The model under review builds one solid part; all positions refer to its coordinate system, in mm. Coordinates: 2 decimals unless noted, no trailing zeros. Loops run counter-clockwise (first coordinate to the right, second up) from the corner with the lowest first, then second, coordinate; pieces in that order, holes last. Notation, with made-up numbers: (17, 89.25) -> (63, 89.25) arc R23 ccw to (63, 118.25) -> close; hole circle Ø11 at (19, -25.75). An arc over 180 degrees is marked (long way). One line per question, with ' | ' between items. Start each with the question number.
from build123d import *

# Parameters (mm, degrees)
F0_W     = 302
F0_H     = 600
F1_DEPTH = 21
F2_SIZE  = 20.99999
F3_W     = 21
F3_H     = 600
F4_DEPTH = 10
F5_W     = 302
F5_H     = 15
F6_DEPTH = 4
F7_W     = 281
F7_H     = 15
F8_DEPTH = 4


# Not quite as in the source:
# - a fillet or chamfer is up to 0.001 mm smaller than in the source, because OpenCascade refuses the exact size


with BuildPart() as f1:
    # F0 (on Front) → F1 (new body)
    with BuildSketch(Plane.XZ):
        with Locations((151, 300)):
            Rectangle(F0_W, F0_H)
    extrude(amount=-F1_DEPTH)

    # F2 (size 21 in the source; OpenCascade refuses exactly that, so slightly less here)
    f2_edges = [f1.edges().sort_by_distance(p)[0] for p in [
        (151, 0, 0),
        (151, 0, 600),
    ]]
    chamfer(f2_edges, length=F2_SIZE)

    # F3 (on face) → F4 (cut)
    with BuildSketch(Plane.XZ):
        with Locations((10.5, 300)):
            Rectangle(F3_W, F3_H)
    extrude(amount=-F4_DEPTH, mode=Mode.SUBTRACT)

    # F5 (on face) → F6 (cut)
    with BuildSketch(Plane.XZ):
        with Locations((151, 507.5)):
            Rectangle(F5_W, F5_H)
    extrude(amount=-F6_DEPTH, mode=Mode.SUBTRACT)

    # F7 (on face) → F8 (cut)
    with BuildSketch(Plane.XZ):
        with Locations((161.5, 335.5)):
            Rectangle(F7_W, F7_H)
        with Locations((161.5, 127.5)):
            Rectangle(F7_W, F7_H)
    extrude(amount=-F8_DEPTH, mode=Mode.SUBTRACT)


solid = f1.part
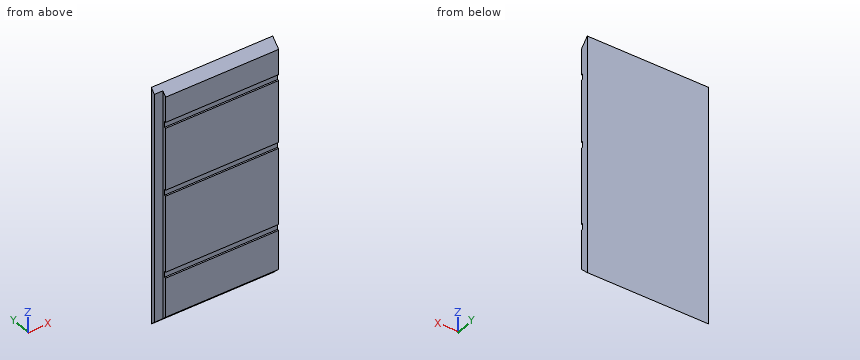
1) Insertion check: pin 1 Ø10 at (x, y) = (209, 10) entering from -Z; pin 2 Ø6 at (x, y) = (64, 17) entering from +Z; pin 3 Ø3 at (x, y) = (209.5, 3) entering from -Z. Each pin has a flat end and moves straight along its axis. Give the tip position at first contact, or say it passes through.
2) Consider section B-B, the plane z = 532. Write out the cut boundary in (x, y).
3) Wall thickness on L1, parallel to X at y = 3, z = 517; L2, parallel to Z at x = 220, y = 10; L3, parallel to Z at x = 272, y = 19.5: over which ranges is each line inside the solid? List them lowest first.
Filled sheet:
1) pin 1: z = 6 | pin 2: z = 599 | pin 3: z = 16.5
2) outline: (0, 10) -> (21, 10) -> (21, 0) -> (302, 0) -> (302, 21) -> (0, 21) -> close
3) L1: 21 to 302 | L2: 11 to 589 | L3: 1.5 to 598.5
